Autodesk Inventor part; units mm, degrees
ref_plane "YZ Plane" through (0, 0, 0) normal (1, 0, 0) x (0, 1, 0)
ref_plane "XZ Plane" through (0, 0, 0) normal (0, 1, 0) x (-1, 0, 0)
ref_plane "XY Plane" through (0, 0, 0) normal (0, 0, 1) x (1, 0, 0)
sketch "Sketch1" plane through (0, 0, 0) normal (0, 0, 1) x (1, 0, 0)
  line L0 (-20, -25) -> (20, -25)
  line L1 (20, -25) -> (20, 25)
  line L2 (20, 25) -> (-20, 25)
  line L3 (-20, 25) -> (-20, -25)
  line L4 (-20, -25) -> (20, 25) construction
  line L5 (20, -25) -> (-20, 25) construction
  point P0 (0, 0)
  dimension "d0" = 40
  dimension "d1" = 50
extrude "Extrusion1" add sketch "Sketch1" along normal blind 5
sketch "Sketch2" plane through (0, 0, 5) normal (0, 0, 1) x (1, 0, 0)
  circle A0 centre (-10, 10) radius 2.5
  circle A1 centre (-10, -10) radius 2.5
  circle A2 centre (10, 10) radius 2.5
  circle A3 centre (10, -10) radius 2.5
  point P0 (0, 0)
  dimension "d4" = 5
  dimension "d5" = 5
  dimension "d6" = 5
  dimension "d7" = 5
  dimension "d8" = 10
  dimension "d9" = 10
  dimension "d10" = 10
  dimension "d11" = 10
extrude "Extrusion2" cut sketch "Sketch2" against normal through all
thread "Thread1"
thread "Thread2"
thread "Thread3"
thread "Thread4"
properties part number "CP010" material "ABS Plastic"
The model under review builds one solid part; all positions refer to its coordinate system, in mm. Give positions to 0.01 mm unless a question says otherwise; leave off trailing zeros. Loops run counter-clockwise (first coordinate to the right, second up) from the corner with the lowest first, then second, coordinate; pieces in that order, holes last. Notation, with made-up numbers: (-1, 51.5) -> (50, 51.5) arc R16 cw to (50, 57.5) -> close; hole circle Ø9 at (58, 86.25). An arc over 180 degrees is marked (long way). Answer as a JSON object with one key per item and string values. Group by question number.
Q1. Draft analysis for pull direction X (two halves, no side actions). For faces 1 (the flat face through (-20, 0, 2)), 2 (the cylindrical face through (-10.54, -12.44, 2.54)), 3 (the cylindrical face through (-10.54, 7.56, 2.54)), 4 (the flat face through (0, 25, 2)), state which applies: pulls with the +X half, pulls with the -X half, needs draft (parallel to the pull), parting line crosses it, or undercut.
Q2. Take a section at B-B (y = 10). Write out the cut boundary in (x, z).
Q3. Insertion check: pin 1 (1.5 mm diameter, centred on x = -13.5, y = 15.5, fed in from -Z). The pin has a flat end and moves straight along its axis. Give the tip position at first contact, or say it passes through.
Q4. Wall thickness on line 1 along Y through (x, z) = (-10, 3.4); line 2 along Y through (x, z) = (10.5, 0.9); line 3 along X through (y, z) = (-10.5, 1.1): over which ranges is each line inside the solid? List them lowest first.
Q5. Take a section at C-C (z = 2.1). Write out the cut boundary in (x, y), plus the area to 3 significant figures.
Q6. Take a section at A-A (x = -10). Write out the cut boundary in (y, z).
Answer below:
{
 "1": {"face 1": "pulls with the -X half", "face 2": "undercut", "face 3": "undercut", "face 4": "needs draft"},
 "2": {"outline": "(-20, 0) -> (-12.5, 0) -> (-12.5, 5) -> (-20, 5) -> close; (-7.5, 0) -> (7.5, 0) -> (7.5, 5) -> (-7.5, 5) -> close; (12.5, 0) -> (20, 0) -> (20, 5) -> (12.5, 5) -> close"},
 "3": {"pin 1": "stops at z = 0"},
 "4": {"line 1": "y = -25 to -12.5, -7.5 to 7.5, 12.5 to 25", "line 2": "y = -25 to -12.45, -7.55 to 7.55, 12.45 to 25", "line 3": "x = -20 to -12.45, -7.55 to 7.55, 12.45 to 20"},
 "5": {"outline": "(-20, -25) -> (20, -25) -> (20, 25) -> (-20, 25) -> close; hole circle Ø5 at (-10, -10); hole circle Ø5 at (-10, 10); hole circle Ø5 at (10, -10); hole circle Ø5 at (10, 10)", "area": "1,920 mm2"},
 "6": {"outline": "(-25, 0) -> (-12.5, 0) -> (-12.5, 5) -> (-25, 5) -> close; (-7.5, 0) -> (7.5, 0) -> (7.5, 5) -> (-7.5, 5) -> close; (12.5, 0) -> (25, 0) -> (25, 5) -> (12.5, 5) -> close"}
}
